Could you check a few things on this drawing? It's one solid part, dimensions in mm from its lowest x, y, z. A direction names the side the tool comes from. Give positions to 0.01 mm unless a question says otherwise; leave off trailing zeros. Order: outer loops, then holes, each group sorted by start corner. A loop starts at its lowest first (then second) coordinate and runs counter-clockwise, first axis right, second up.
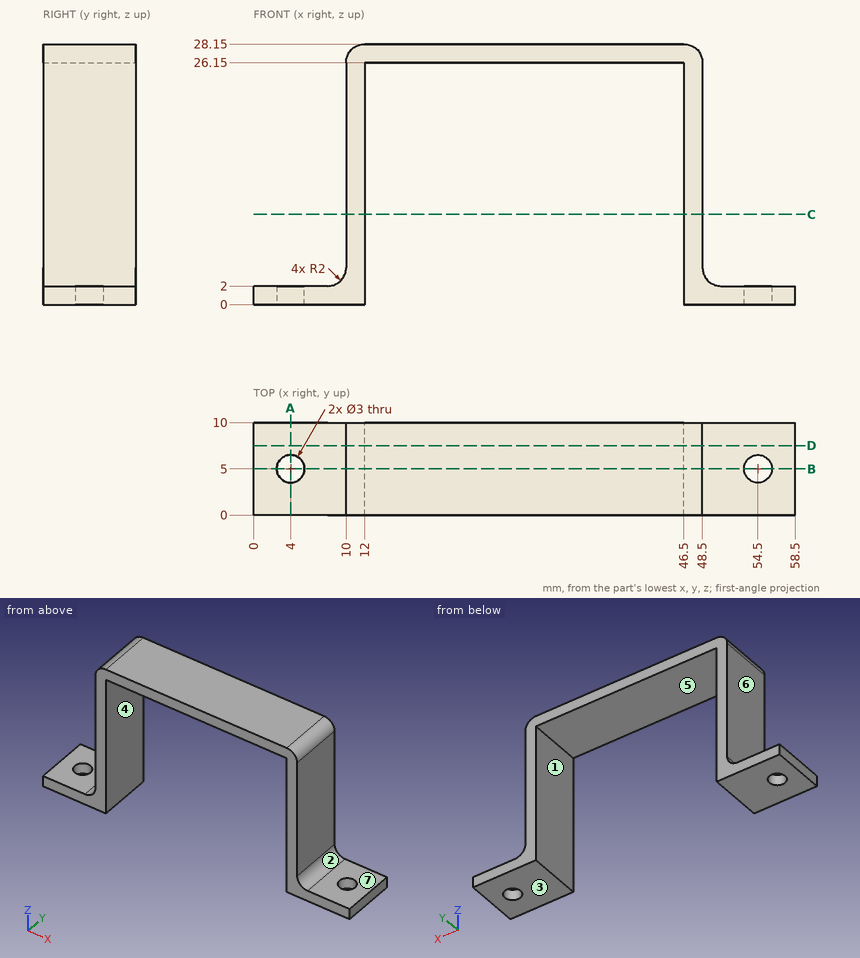
1) Suppose I cut it at B-B (y = 5). Please give me the cut outline in (x, z), and give its area (3 significant figures).
2) I'm going to push a flat-ended pin straight in: pin 1 Ø4 at (x, y) = (6, 3) entering from +Z. Where does the tip first touch, or does it pass through?
3) Suppose I cut it at C-C (z = 9.75). Please give me the cut outline in (x, y), and give its area (3 significant figures).
4) If I drill on line 1 (X direction, y = 2.25, z = 10.75); line 2 (Y direction, x = 4, z = 1.5); line 3 (Z direction, x = 14, y = 7), over which ranges is the centre line in solid material (lowest first)?
5) Which directions (+Z, -Z, +X, -X, +Y, -Y) give clear straight access to the entire face, cutting with the end or side of a thin tool? Please do the marked faces 5, 6 and 7.
6) We'd pull the mould along X, two halves only. Please class the marked faces 1, 2, 3 and 4: +X half, -X half, draft (parallel to the pull), parting line (faces both ways), or undercut.
7) Suppose I cut it at D-D (y = 7.5). Please give me the cut outline in (x, z), and give its area (3 significant figures).
8) Suppose I cut it at A-A (x = 4). Please give me the cut outline in (y, z).
Results:
1. outline: (0, 0) - (2.5, 0) - (2.5, 2) - (0, 2) - close; (5.5, 0) - (12, 0) - (12, 26.15) - (46.5, 26.15) - (46.5, 0) - (53, 0) - (53, 2) - (50.5, 2) arc R2 cw to (48.5, 4) - (48.5, 26.15) arc R2 ccw to (46.5, 28.15) - (12, 28.15) arc R2 ccw to (10, 26.15) - (10, 4) arc R2 cw to (8, 2) - (5.5, 2) - close; (56, 0) - (58.5, 0) - (58.5, 2) - (56, 2) - close
1. area: 210 mm2
2. pin 1: stops at z = 2
3. outline: (10, 0) - (12, 0) - (12, 10) - (10, 10) - close; (46.5, 0) - (48.5, 0) - (48.5, 10) - (46.5, 10) - close
3. area: 40.0 mm2
4. line 1: x = 10 to 12, 46.5 to 48.5
4. line 2: y = 0 to 3.5, 6.5 to 10
4. line 3: z = 26.15 to 28.15
5. face 5: -Z, +Y, -Y
5. face 6: +Z, -X, +Y, -Y
5. face 7: +Z, +X, +Y, -Y
6. face 1: undercut
6. face 2: +X half
6. face 3: draft
6. face 4: undercut
7. outline: (0, 0) - (12, 0) - (12, 26.15) - (46.5, 26.15) - (46.5, 0) - (58.5, 0) - (58.5, 2) - (50.5, 2) arc R2 cw to (48.5, 4) - (48.5, 26.15) arc R2 ccw to (46.5, 28.15) - (12, 28.15) arc R2 ccw to (10, 26.15) - (10, 4) arc R2 cw to (8, 2) - (0, 2) - close
7. area: 222 mm2
8. outline: (0, 0) - (3.5, 0) - (3.5, 2) - (0, 2) - close; (6.5, 0) - (10, 0) - (10, 2) - (6.5, 2) - close
